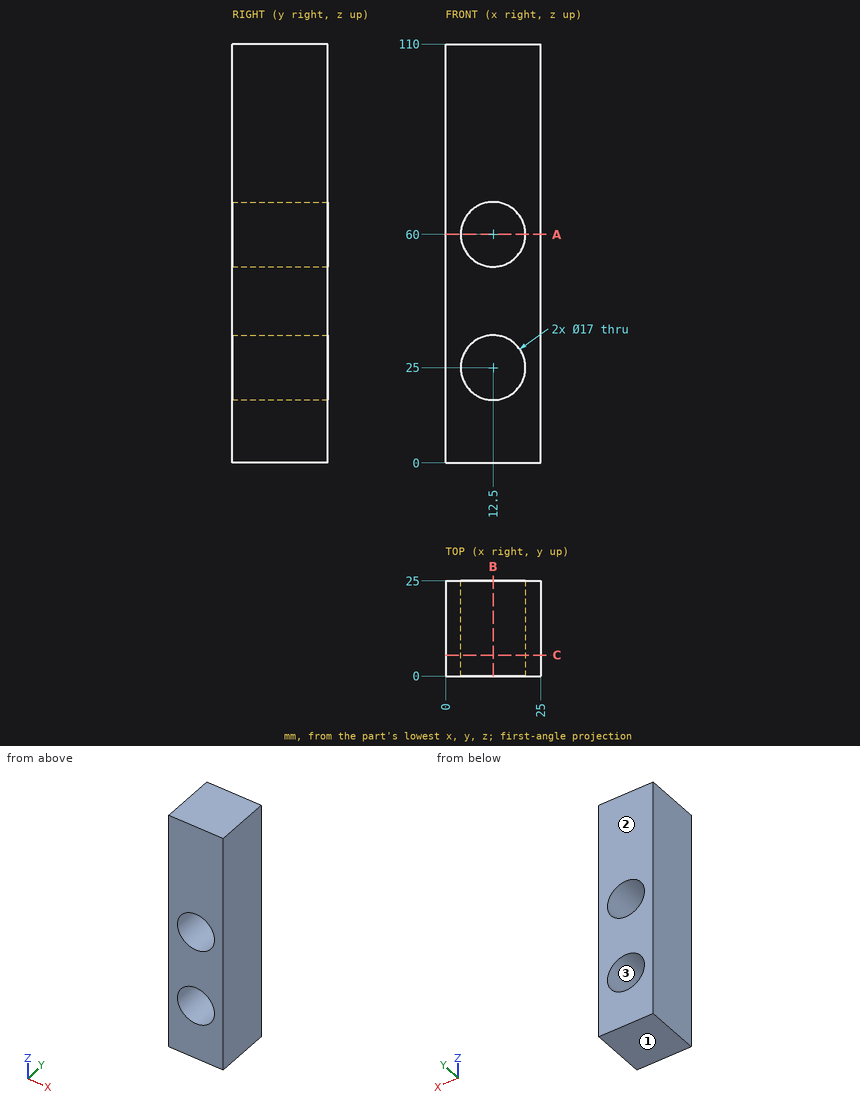
Part print with two shaded views. Sizes in mm from the minimum x, y, z corner. Round coordinates to 2 decimals unless told otherwise and drop trailing zeros. Write each loop counter-clockwise with the first axis right and the second up, starting at its lowest first coordinate (ties: lowest second). Pieces come first, ordered by that corner, then holes. Notation, with made-up numbers: (39, 64.5) -> (92, 64.5) arc R22 ccw to (92, 71.5) -> close; hole circle Ø5 at (-34, -10). An arc over 180 degrees is marked (long way). Use one line per item in the form item = value.
Q1. Band-saw the part on C-C, the plane y = 5.5. Write the cut outline in (x, z).
Conclusion:
outline = (0, 0) -> (25, 0) -> (25, 110) -> (0, 110) -> close; hole circle Ø17 at (12.5, 25); hole circle Ø17 at (12.5, 60)
Q2. Band-saw the part on A-A, the plane z = 60. Write the cut outline in (x, y), then the cut area to 3 significant figures.
Conclusion:
outline = (0, 0) -> (4, 0) -> (4, 25) -> (0, 25) -> close; (21, 0) -> (25, 0) -> (25, 25) -> (21, 25) -> close
area = 200 mm²
Q3. Drop a flat-ended pin along its axis: P1, Ø6, axis at x = 19.5, y = 12, coming from the -Z side. Give the stop position or say it passes through.
Conclusion:
P1 = 0
Q4. Band-saw the part on B-B, the plane x = 12.5. Write the cut outline in (y, z), then the cut area to 3 significant figures.
Conclusion:
outline = (0, 0) -> (25, 0) -> (25, 16.5) -> (0, 16.5) -> close; (0, 33.5) -> (25, 33.5) -> (25, 51.5) -> (0, 51.5) -> close; (0, 68.5) -> (25, 68.5) -> (25, 110) -> (0, 110) -> close
area = 1,900 mm²
Q5. Drill centre lines: L1, parallel to Z at x = 12.75, y = 20.5; L2, parallel to Z at x = 15.75, y = 14.5; L3, parallel to X at y = 10.25, z = 64. Where is each one in solid material? Low to high.
Conclusion:
L1 = 0 to 16.5, 33.5 to 51.5, 68.5 to 110
L2 = 0 to 17.15, 32.85 to 52.15, 67.85 to 110
L3 = 0 to 5, 20 to 25
Q6. Two-plate mould, pull along Z, no slides. Class the marked faces 1, 2 and 3: released by +Z, released by -Z, zero draft, split by the parting line, or undercut.
Conclusion:
face_1 = released by -Z
face_2 = zero draft
face_3 = undercut
